Read the model definition and answer for the solid it produces. Units are mm, in the model's axes. A direction names the side the tool comes from. Give positions to 0.01 mm unless a question says otherwise; leave off trailing zeros. Write each loop counter-clockwise with the first axis right and the second up, starting at its lowest first coordinate (ties: lowest second). Pieces come first, ordered by that corner, then holes. Notation, with made-up numbers: (38.25, -11.5) - (62.25, -11.5) arc R29 cw to (62.25, 14.5) - close; hole circle Ø6 at (-15, 23.25). An arc over 180 degrees is marked (long way). Use CSV: the item, a comma, the result in double quotes. Start each with the question number.
from build123d import *

# Parameters (mm, degrees)
EXTRUDE_1_DEPTH     = 26.5
SKETCH_4_R          = 4.8
SKETCH_4_R_2        = 1.6
CUT_EXTRUDE_1_DEPTH = 26
SKETCH_5_R          = 1.6
CUT_EXTRUDE_2_DEPTH = 26
SKETCH_6_R          = 12.95
EXTRUDE_2_DEPTH     = 48
EXTRUDE_START       = 14
SKETCH_7_R          = 4
EXTRUDE_3_DEPTH     = 14


with BuildPart() as part:
    # 草图2 → 凸台-拉伸1 (new body)
    with BuildSketch(Plane(origin=(0, 0, 0), x_dir=(1, 0, 0), z_dir=(0, 1, 0))):
        with BuildLine():
            Line((-23.472034258, 6.497634693), (-23.472034258, 3.497634693))
            Line((-23.472034258, 3.497634693), (4.527965742, 3.497634693))
            ThreePointArc((4.527965742, 3.497634693), (5.942179305, 2.911848255), (6.527965742, 1.497634693))
            Line((6.527965742, 1.497634693), (6.527965742, -26.502365307))
            Line((6.527965742, -26.502365307), (9.527965742, -26.502365307))
            Line((9.527965742, -26.502365307), (9.527965742, 4.497634693))
            ThreePointArc((9.527965742, 4.497634693), (8.942179305, 5.911848255), (7.527965742, 6.497634693))
            Line((7.527965742, 6.497634693), (-23.472034258, 6.497634693))
        make_face()
    extrude(amount=EXTRUDE_1_DEPTH)

    # 草图4 → 切除-拉伸1 (cut)
    with BuildSketch(Plane(origin=(0, 0, -6.497634693), x_dir=(-1, 0, 0), z_dir=(0, 0, -1))):
        with Locations((6.972034258, 13.25)):
            Circle(SKETCH_4_R)
        with Locations((-0.244612027, 21.054928982)):
            Circle(SKETCH_4_R_2)
        with Locations((14.788478141, 21.054928982)):
            Circle(SKETCH_4_R_2)
        with Locations((14.788478141, 6.021838814)):
            Circle(SKETCH_4_R_2)
        with Locations((-0.244612027, 6.021838814)):
            Circle(SKETCH_4_R_2)
    extrude(amount=-CUT_EXTRUDE_1_DEPTH, mode=Mode.SUBTRACT)

    # 草图5 → 切除-拉伸2 (cut)
    with BuildSketch(Plane(origin=(9.527965742, 0, 0), x_dir=(0, 0, -1), z_dir=(1, 0, 0))):
        with BuildLine():
            Line((-26.502365307, 26.5), (-26.502365307, 0))
            Line((-26.502365307, 0), (-11.002365307, 0))
            ThreePointArc((-11.002365307, 0), (-24.252365307, 13.25), (-11.002365307, 26.5))
            Line((-11.002365307, 26.5), (-26.502365307, 26.5))
        make_face()
        with BuildLine():
            Line((-11.002365307, 9.25), (-1.637230429, 9.25))
            ThreePointArc((-1.637230429, 9.25), (2.362769571, 13.25), (-1.637230429, 17.25))
            Line((-1.637230429, 17.25), (-11.002365307, 17.25))
            ThreePointArc((-11.002365307, 17.25), (-15.002365307, 13.25), (-11.002365307, 9.25))
        make_face()
        with Locations((-11.002365307, 4.75)):
            Circle(SKETCH_5_R)
        with Locations((-11.002365307, 21.75)):
            Circle(SKETCH_5_R)
    extrude(amount=-CUT_EXTRUDE_2_DEPTH, mode=Mode.SUBTRACT)

    # 草图6 → 凸台-拉伸2 (add)
    with BuildSketch(Plane.ZY.offset(-6.527965742)):
        with Locations(Location((11.002365307, 13.25, 0), (0, 0, 170.757909694))):
            Circle(SKETCH_6_R)
    extrude(amount=EXTRUDE_2_DEPTH)

    # 草图7 → 凸台-拉伸3 (add)
    with BuildSketch(Plane(origin=(6.527965742, 0, 0), x_dir=(0, 0, -1), z_dir=(1, 0, 0)).offset(EXTRUDE_START)):
        with Locations(Location((-11.002365307, 13.25, 0), (0, 0, 270))):
            Circle(SKETCH_7_R)
    extrude(amount=-EXTRUDE_3_DEPTH)


solid = part.part
(1) The part is cut by section A-A on y = 13.25. Write down the section's boundary in (x, z).
(2) Given P1, Ø2, axis at x = -18.5, z = 15.5, coming from the -Y side; P2, Ø1, axis at y = 4.5, z = 11, coming from the +X side; P3, Ø4, axis at y = 6, z = -0.5, coming from the +X side, each flat-ended and moving along its own axis, determine where each tip first touches the part or whether it passes through.
(3) Consider probe 1 along X at (y, z) = (2.5, 3); probe 2 along X at (y, z) = (19, 19); probe 3 along Z at (x, y) = (-6.5, 23.75). Determine where each line is inside the solid, lowest interval first.
(4) Which of the six approach directions +Z, -Z, +X, -X, +Y, -Y give full straight-line access (tool end or side, diameter ignored) to faces 4 (the face through (-17.1, 19.4, 22.4)), 5 (the face through (6.528, 14, 3)), 6 (the face through (-15.6, 7.4, -5)), 7 (the face through (-13, 13, -3.498))?
(5) The part is cut by section D-D on z = 17. Write down the section's boundary in (x, y), plus the area to 3 significant figures.
(6) The part is cut by section C-C on x = 2.5. Write down the section's boundary in (y, z).
(7) For a pull along X with two mould halves and no side action, classify faces 1 (the face through (5.927, 13.064, -2.927)), 2 (the face through (20.528, 13, 11)), 3 (the face through (-15.527, 19.635, -5.019)) as pulls with the +X half, pulls with the -X half, needs draft (parallel to the pull), parting line crosses it, or undercut.
(8) The part is cut by section B-B on x = -10.5. Write down the section's boundary in (y, z).
Reported:
1,outline,"(-41.47, -1.95) - (6.53, -1.95) - (6.53, 7) - (20.53, 7) - (20.53, 15) - (9.53, 15) - (9.53, 24.25) - (6.53, 24.25) - (6.53, 23.95) - (-41.47, 23.95) - close; (-23.47, -6.5) - (-11.77, -6.5) - (-11.77, -3.5) - (-23.47, -3.5) - close; (-2.17, -6.5) - (7.53, -6.5) arc R2 ccw to (9.53, -4.5) - (9.53, -2.36) - (6.33, -2.36) arc R2 cw to (4.53, -3.5) - (-2.17, -3.5) - close"
2,P1,"y = 0.78"
2,P2,"x = 6.53"
2,P3,"x = 9.53"
3,probe 1,"6.53 to 9.53"
3,probe 2,"-41.47 to 9.53"
3,probe 3,"-6.5 to -3.5, 3.42 to 18.58"
4,face 4,"-X"
4,face 5,"+X"
4,face 6,"-Z"
4,face 7,"-X, +Y, -Y"
5,outline,"(-41.47, 1.77) - (6.53, 1.77) - (6.53, 1.44) - (9.53, 1.44) - (9.53, 25.06) - (6.53, 25.06) - (6.53, 24.73) - (-41.47, 24.73) - close"
5,area,"1,170 mm²"
6,outline,"(0, -6.5) - (26.5, -6.5) - (26.5, -3.5) - (0, -3.5) - close; circle Ø25.9 at (13.25, 11)"
7,face 1,"pulls with the -X half"
7,face 2,"pulls with the +X half"
7,face 3,"undercut"
8,outline,"(0, -6.5) - (10, -6.5) - (10, -3.5) - (0, -3.5) - close; circle Ø25.9 at (13.25, 11); (16.5, -6.5) - (26.5, -6.5) - (26.5, -3.5) - (16.5, -3.5) - close"
